```python
from build123d import *

# Parameters (mm, degrees)
F0_R     = 43.957612
F1_DEPTH = 132.08


with BuildPart() as f1:
    # F0 (on Front) → F1 (new body)
    with BuildSketch(Plane.XZ):
        Polygon((-35.785236, 52.508596), (-63.364603, 4.76055), (-43.229131, -46.572287), (9.458758, -62.835242), (55.024009, -31.781978), (59.155059, 23.203763), (18.741144, 60.716598), align=None)
        Circle(F0_R, mode=Mode.SUBTRACT)
    extrude(amount=F1_DEPTH)


solid = f1.part
```
Geometry: final body of the model. Coordinates: model frame, mm. Round coordinates to 2 decimals unless told otherwise and drop trailing zeros. Write each loop counter-clockwise with the first axis right and the second up, starting at its lowest first coordinate (ties: lowest second). Pieces come first, ordered by that corner, then holes. Notation, with made-up numbers: (86.25, -16.75) -> (99.25, -16.75) arc R31 cw to (99.25, 12.25) -> close; hole circle Ø11 at (-30.75, 4). An arc over 180 degrees is marked (long way). Return JSON: item names as keys, results as strings.
Q1. First-contact query: pin 1 Ø12 at (y, z) = (-60, 10.5) entering from -X; pin 2 Ø10 at (x, y) = (41, -98.5) entering from +Z; pin 3 Ø5 at (y, z) = (-43, -23) entering from +X. Flat tips, straight axial feed; report the tip coordinate or a pass-through.
From the geometry:
{"pin 1": "x = -63.36", "pin 2": "z = 44.7", "pin 3": "x = 55.87"}
Q2. Mould query, pull axis X, two halves, no side actions, for faces 1 (the flat face through (31.92, -65.12, -47.53)), 2 (the cylindrical face through (40.606, -65.115, -16.836)), 3 (the flat face through (-34.2, -132.08, -28.2)). Classes: +X half, -X half, draft (parallel to the pull), parting line (faces both ways), or undercut.
From the geometry:
{"face 1": "+X half", "face 2": "undercut", "face 3": "draft"}
Q3. Ray query, line 1 (X direction, y = -107, z = 20); line 2 (X direction, y = -125, z = 27); line 3 (Z direction, x = 0, y = -89). Return the intervals inside material, ascending.
From the geometry:
{"line 1": "-54.56 to -39.14, 39.14 to 58.91", "line 2": "-50.52 to -34.69, 34.69 to 55.07", "line 3": "-59.92 to -43.96, 43.96 to 57.9"}
Q4. Section C-C on z = 21. Return the cut outline in (x, y), and give its area (3 significant figures).
From the geometry:
{"outline": "(-53.98, -132.08) -> (-38.62, -132.08) -> (-38.62, 0) -> (-53.98, 0) -> close; (38.62, -132.08) -> (58.99, -132.08) -> (58.99, 0) -> (38.62, 0) -> close", "area": "4,720 mm2"}
Q5. Section A-A on x = 23.5. Return the cut outline in (y, z).
From the geometry:
{"outline": "(-132.08, -53.27) -> (0, -53.27) -> (0, -37.15) -> (-132.08, -37.15) -> close; (-132.08, 37.15) -> (0, 37.15) -> (0, 56.3) -> (-132.08, 56.3) -> close"}
Q6. Section D-D on z = -51. Return the cut outline in (x, y).
From the geometry:
{"outline": "(-28.88, -132.08) -> (26.82, -132.08) -> (26.82, 0) -> (-28.88, 0) -> close"}
Q7. Section B-B on y = -78.5. Return the cut outline in (x, z), and give its area (3 significant figures).
From the geometry:
{"outline": "(-63.36, 4.76) -> (-43.23, -46.57) -> (9.46, -62.84) -> (55.02, -31.78) -> (59.16, 23.2) -> (18.74, 60.72) -> (-35.79, 52.51) -> close; hole circle Ø87.92 at (0, 0)", "area": "4,980 mm2"}
